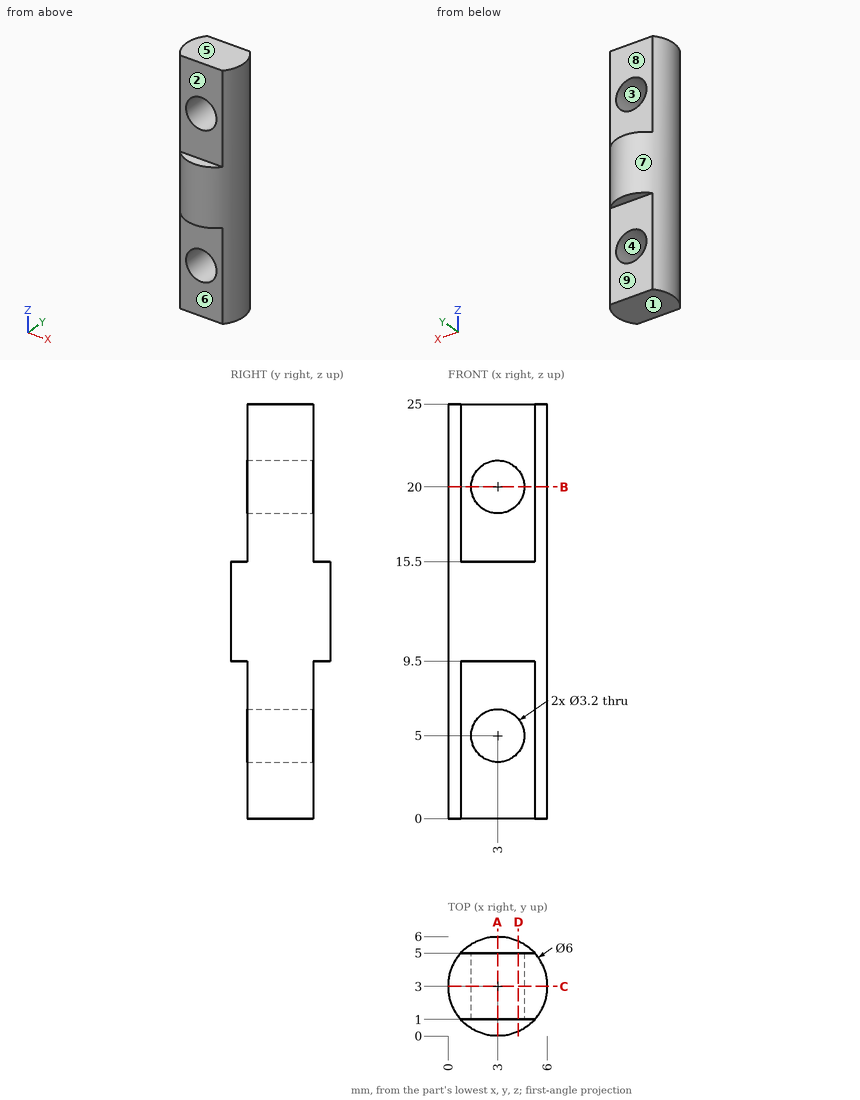
For this review, use the dimensioned drawing (mm, ordinates from the lowest corner) and the shaded views. A direction names the side the tool comes from. Give positions to 0.01 mm unless a question says otherwise; leave off trailing zeros. Write each loop counter-clockwise with the first axis right and the second up, starting at its lowest first coordinate (ties: lowest second). Pieces come first, ordered by that corner, then holes. Notation, with made-up numbers: M -0.5,69 L 52.5,69 A23 ccw 52.5,95 Z; hole C -16.5,68 d5. An arc over 180 degrees is marked long. Write item = value, one per line. Start each with the question number.
Q1. Mouldability with a two-part tool opening along Z and no side actions: class the marked faces 1, 2, 3 and 4 as released by +Z, released by -Z, zero draft, split by the parting line, or undercut.
Q2. We need section A-A (x = 3). State the section outline as (y, z) points, plus the area to 3 significant figures.
Q3. Clearance check with flat-ended pins moving along their axes: pin 1 (1.5 mm diameter, centred on x = 2, z = 6, fed in from -Y); pin 2 (3.5 mm diameter, centred on x = 2, z = 18, fed in from +Y); pin 3 (3 mm diameter, centred on x = 3, z = 20, fed in from +Y); pin 4 (0.5 mm diameter, centred on x = 3.5, y = 5.5, fed in from +Z). State where each tip first meets the part, or that it passes through.
Q4. We need section B-B (z = 20). State the section outline as (x, y) points.
Q5. Machinability: for the marked faces 5, 6, 7, 8 and 9, which of the approach directions +Z, -Z, +X, -X, +Y, -Y give a long, thin tool a straight path to every point of the face, cutting with its end or side? Answer none if there is none.
Q6. For line 1 (Z direction, x = 3, y = 3.25); line 2 (Z direction, x = 2.1, y = 4.55); line 3 (Y direction, x = 5.15, z = 21), list the stretches that pass through material, from the lowest coordinate up.
Q7. We need section C-C (y = 3). State the section outline as (x, z) points, plus the area to 3 significant figures.
Q8. We need section D-D (x = 4.25). State the section outline as (y, z) points.
Result set:
q1.face_1 = released by -Z
q1.face_2 = zero draft
q1.face_3 = undercut
q1.face_4 = undercut
q2.outline = M 0,9.5 L 1,9.5 L 1,6.6 L 5,6.6 L 5,9.5 L 6,9.5 L 6,15.5 L 5,15.5 L 5,18.4 L 1,18.4 L 1,15.5 L 0,15.5 Z; M 1,0 L 5,0 L 5,3.4 L 1,3.4 Z; M 1,21.6 L 5,21.6 L 5,25 L 1,25 Z
q2.area = 86.4 mm2
q3.pin_1 = 1
q3.pin_2 = 5
q3.pin_3 = through
q3.pin_4 = 15.5
q4.outline = M 0.76,1 L 1.4,1 L 1.4,5 L 0.76,5 A3 ccw Z; M 4.6,1 L 5.24,1 A3 ccw 5.24,5 L 4.6,5 Z
q5.face_5 = +Z, +X, -X, +Y, -Y
q5.face_6 = -Z, +X, -X, -Y
q5.face_7 = +Z, -Z
q5.face_8 = +Z, +X, -X, +Y
q5.face_9 = -Z, +X, -X, +Y
q6.line_1 = 0 to 3.4, 6.6 to 18.4, 21.6 to 25
q6.line_2 = 0 to 3.68, 6.32 to 18.68, 21.32 to 25
q6.line_3 = 1 to 5
q7.outline = M 0,0 L 6,0 L 6,25 L 0,25 Z; hole C 3,5 d3.2; hole C 3,20 d3.2
q7.area = 134 mm2
q8.outline = M 0.27,9.5 L 1,9.5 L 1,6 L 5,6 L 5,9.5 L 5.73,9.5 L 5.73,15.5 L 5,15.5 L 5,19 L 1,19 L 1,15.5 L 0.27,15.5 Z; M 1,0 L 5,0 L 5,4 L 1,4 Z; M 1,21 L 5,21 L 5,25 L 1,25 Z
